Answer from the drawing. Dimensions are ordinates in mm from the lowest x, y and z of the part. Round coordinates to 2 decimals unless told otherwise and drop trailing zeros. Order: outer loops, then holes, each group sorted by start corner. A loop starts at its lowest first (then second) coordinate and runs counter-clockwise, first axis right, second up. Notation, with made-up numbers: (70, 46.25) -> (79, 46.25) arc R34 ccw to (79, 76.25) -> close; hole circle Ø10 at (72.5, 16.5). An arc over 180 degrees is marked (long way). Use a Markdown table: item, result. Add a question column.
1. The mould has two halves that part along Y. Classify the marked faces 1, 2, 3 and 4: +Y half, -Y half, draft (parallel to the pull), parting line (faces both ways), or undercut.
2. Section C-C, the plane y = 32 is taken. Give the vertices of the cut face in (x, z), then the cut area to 3 significant figures.
3. Consider L1, parallel to Y at x = 12, z = 3.1; L2, parallel to Y at x = 2, z = 3.2; L3, parallel to X at y = 48, z = 4.3. Determine where each line is inside the solid, lowest interval first. Write a range as [from, to].
4. Given pin 1 (1.8 mm diameter, centred on x = 12, y = 32, fed in from +Z), flat-ended and moving along its own axis, determine where the tip first touches the part or whether it passes through.
5. Section D-D, the plane x = 15.25 is taken. Give the vertices of the cut face in (y, z), then the cut area to 3 significant figures.
6. Section A-A, the plane x = 4 is taken. Give the vertices of the cut face in (y, z), then the cut area to 3 significant figures.
7. Section B-B, the plane z = 3 is taken. Give the vertices of the cut face in (x, y).
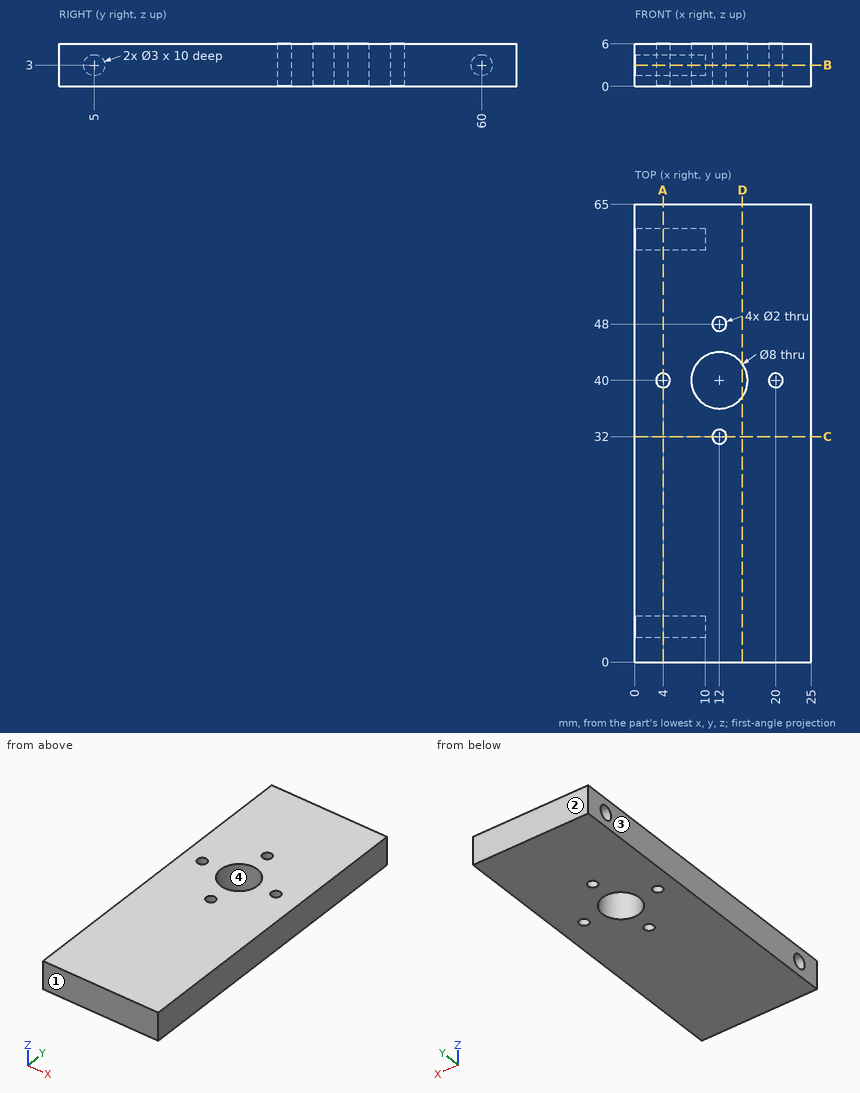
Verdict:
| question | item | result |
|---|---|---|
| 1 | face 1 | -Y half |
| 1 | face 2 | +Y half |
| 1 | face 3 | draft |
| 1 | face 4 | undercut |
| 2 | outline | (0, 0) -> (11, 0) -> (11, 6) -> (0, 6) -> close; (13, 0) -> (25, 0) -> (25, 6) -> (13, 6) -> close |
| 2 | area | 138 mm2 |
| 3 | L1 | y = [0, 31], [33, 36], [44, 47], [49, 65] |
| 3 | L2 | y = [0, 3.51], [6.49, 58.51], [61.49, 65] |
| 3 | L3 | x = [0, 11], [13, 25] |
| 4 | pin 1 | passes through |
| 5 | outline | (0, 0) -> (37.67, 0) -> (37.67, 6) -> (0, 6) -> close; (42.33, 0) -> (65, 0) -> (65, 6) -> (42.33, 6) -> close |
| 5 | area | 362 mm2 |
| 6 | outline | (0, 0) -> (39, 0) -> (39, 6) -> (0, 6) -> close; (41, 0) -> (65, 0) -> (65, 6) -> (41, 6) -> close; hole circle Ø3 at (5, 3); hole circle Ø3 at (60, 3) |
| 6 | area | 364 mm2 |
| 7 | outline | (0, 0) -> (25, 0) -> (25, 65) -> (0, 65) -> (0, 61.5) -> (10, 61.5) -> (10, 58.5) -> (0, 58.5) -> (0, 6.5) -> (10, 6.5) -> (10, 3.5) -> (0, 3.5) -> close; hole circle Ø2 at (4, 40); hole circle Ø8 at (12, 40); hole circle Ø2 at (12, 32); hole circle Ø2 at (12, 48); hole circle Ø2 at (20, 40) |
